Design review of the part built by this model. Coordinates are the model's own, in mm. A direction names the side the tool comes from. Coordinates: 2 decimals unless noted, no trailing zeros. Order: outer loops, then holes, each group sorted by start corner. A loop starts at its lowest first (then second) coordinate and runs counter-clockwise, first axis right, second up.
from build123d import *

# Parameters (mm, degrees)
CHANFREIN1_SIZE              = 0.5
CONG_1_R                     = 0.5
ENL_V_MAT_EXTRU_1_DEPTH      = 22.901027373
ENL_V_MAT_EXTRU_1_DEPTH_BACK = 22.901027373
ESQUISSE2_W                  = 1.8
ESQUISSE2_H                  = 1.4


with BuildPart() as part:
    # Esquisse1 → Révolution1 (revolve)
    with BuildSketch(Plane.XY, mode=Mode.PRIVATE) as r_volution1_sk:
        Polygon((0, 0), (0, 2), (-18, 2), (-18, 2.95), (-21.5, 2.95), (-21.5, 0), align=None)
    revolve(r_volution1_sk.sketch.rotate(Axis((-6, 0, 0), (1, 0, 0)), 90), axis=Axis((-6, 0, 0), (1, 0, 0)))

    # Chanfrein1
    chanfrein1_edges = [part.edges().sort_by_distance(p)[0] for p in [
        (0, 0, -2),
    ]]
    chamfer(chanfrein1_edges, length=CHANFREIN1_SIZE)

    # Congé1
    cong_1_edges = [part.edges().sort_by_distance(p)[0] for p in [
        (-21.5, 0, -2.95),
    ]]
    fillet(cong_1_edges, radius=CONG_1_R)

    # Esquisse2 → Enlèv. mat.-Extru.1 (cut, two sides: drawn at the far end of the back side and taken through both)
    with BuildSketch(Plane.XY.offset(-ENL_V_MAT_EXTRU_1_DEPTH_BACK)):
        with Locations((-20.6, 0)):
            Rectangle(ESQUISSE2_W, ESQUISSE2_H)
    extrude(amount=ENL_V_MAT_EXTRU_1_DEPTH + ENL_V_MAT_EXTRU_1_DEPTH_BACK, mode=Mode.SUBTRACT)


solid = part.part
1. Add section C-C (x = -19). Give the boundary of the cut face in (y, z).
2. Add section B-B (y = 0). Give the boundary of the cut face in (x, z).
3. For faces 1 (the flat face through (-21, -0.7, 0)), 2 (the flat face through (-21.5, -1, 0)), 3 (the cylindrical face through (-9, 2, 0)), list the 3-axis set-ups (+Z, -Z, +X, -X, +Y, -Y) from which the entire face can be reached by the end or side of a thin tool; tool diameter is ignored.
4. Add section A-A (z = 0). Give the boundary of the cut face in (x, y).
5. Insertion check: pin 1 (3 mm diameter, centred on x = -8.5, z = -1, fed in from +Y); pin 2 (0.9 mm diameter, centred on x = -21, z = 0.5, fed in from -Y); pin 3 (1 mm diameter, centred on x = -7.5, z = -0.5, fed in from -Y). Each pin has a flat end and moves straight along its axis. Give the tip position at first contact, or say it passes through.
6. Add section D-D (x = -6). Give the boundary of the cut face in (y, z).
7. To check wall thickness, follow line 1 (X direction, y = -1.45, z = 1.75); line 2 (X direction, y = 0.35, z = 0); line 3 (Y direction, x = -17.25, z = 0.05). State the ranges of each line that lie inside material, in increasing order.
Solution:
1. outline: circle Ø5.9 at (0, 0)
2. outline: (-19.7, -2.95) - (-18, -2.95) - (-18, -2) - (-0.5, -2) - (0, -1.5) - (0, 1.5) - (-0.5, 2) - (-18, 2) - (-18, 2.95) - (-19.7, 2.95) - close
3. face 1: +Z, -Z, -X
3. face 2: +Z, -Z, -X, +Y, -Y
3. face 3: +X
4. outline: (-21.5, -2.45) arc R0.5 ccw to (-21, -2.95) - (-18, -2.95) - (-18, -2) - (-0.5, -2) - (0, -1.5) - (0, 1.5) - (-0.5, 2) - (-18, 2) - (-18, 2.95) - (-21, 2.95) arc R0.5 ccw to (-21.5, 2.45) - (-21.5, 0.7) - (-19.7, 0.7) - (-19.7, -0.7) - (-21.5, -0.7) - close
5. pin 1: stops at y = 2
5. pin 2: stops at y = -2.95
5. pin 3: stops at y = -2
6. outline: circle Ø4 at (0, 0)
7. line 1: x = -21.5 to -18
7. line 2: x = -19.7 to 0
7. line 3: y = -2 to 2
